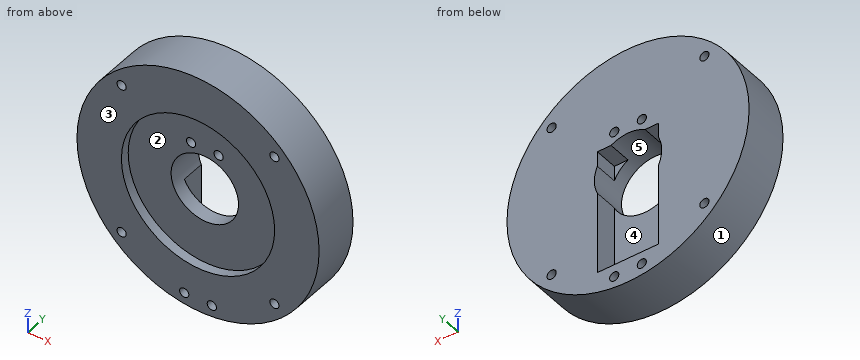
from build123d import *

# Parameters (mm, degrees)
CROQUIS1_R              = 39.5
CROQUIS1_R_2            = 11
CROQUIS1_R_3            = 1.5
SALIENTE_EXTRUIR2_DEPTH = 15
CROQUIS2_R              = 1.5
CROQUIS2_W              = 20
CROQUIS2_H              = 41
CORTAR_EXTRUIR1_DEPTH   = 7.5
CROQUIS2_2_R            = 1.5
CORTAR_EXTRUIR2_DEPTH   = 16
CROQUIS3_R              = 25
CORTAR_EXTRUIR3_DEPTH   = 3


with BuildPart() as part:
    # Croquis1 → Saliente-Extruir2 (new body)
    with BuildSketch(Plane(origin=(0, 0, 0), x_dir=(1, 0, 0), z_dir=(0, 1, 0))):
        Circle(CROQUIS1_R)
        Circle(CROQUIS1_R_2, mode=Mode.SUBTRACT)
        with Locations((24.925514037, 24.925514037)):
            Circle(CROQUIS1_R_3, mode=Mode.SUBTRACT)
        with Locations((24.925514037, -24.925514037)):
            Circle(CROQUIS1_R_3, mode=Mode.SUBTRACT)
        with Locations((-24.925514037, -24.925514037)):
            Circle(CROQUIS1_R_3, mode=Mode.SUBTRACT)
        with Locations((-24.925514037, 24.925514037)):
            Circle(CROQUIS1_R_3, mode=Mode.SUBTRACT)
    extrude(amount=SALIENTE_EXTRUIR2_DEPTH)

    # Croquis2 → Cortar-Extruir1 (cut)
    with BuildSketch(Plane(origin=(0, 15, 0), x_dir=(1, 0, 0), z_dir=(0, 1, 0))):
        with Locations((-4.5, -13.5)):
            Circle(CROQUIS2_R)
        with Locations((4.5, -13.5)):
            Circle(CROQUIS2_R)
        with Locations((4.5, 35.5)):
            Circle(CROQUIS2_R)
        with Locations((-4.5, 35.5)):
            Circle(CROQUIS2_R)
        with Locations((0, 11)):
            Rectangle(CROQUIS2_W, CROQUIS2_H)
    extrude(amount=-CORTAR_EXTRUIR1_DEPTH, mode=Mode.SUBTRACT)

    # Croquis2<2> → Cortar-Extruir2 (cut, through all)
    with BuildSketch(Plane(origin=(0, 15, 0), x_dir=(1, 0, 0), z_dir=(0, 1, 0))):
        with Locations((-4.5, 35.5)):
            Circle(CROQUIS2_2_R)
        with Locations((4.5, 35.5)):
            Circle(CROQUIS2_2_R)
        with Locations((4.5, -13.5)):
            Circle(CROQUIS2_2_R)
        with Locations((-4.5, -13.5)):
            Circle(CROQUIS2_2_R)
    extrude(amount=-CORTAR_EXTRUIR2_DEPTH, mode=Mode.SUBTRACT)

    # Croquis3 → Cortar-Extruir3 (cut)
    with BuildSketch(Plane.XZ):
        Circle(CROQUIS3_R)
    extrude(amount=-CORTAR_EXTRUIR3_DEPTH, mode=Mode.SUBTRACT)


solid = part.part
The listing builds one solid part. Answer for the finished solid, in the listing's coordinates (mm). Face numbers are marked on the shaded views. A direction names the side the tool comes from. Coordinates: 2 decimals unless noted, no trailing zeros. Write each loop counter-clockwise with the first axis right and the second up, starting at its lowest first coordinate (ties: lowest second). Pieces come first, ordered by that corner, then holes. Notation, with made-up numbers: (12.5, -15.75) -> (66.5, -15.75) arc R21 ccw to (66.5, 6.25) -> close; hole circle Ø10 at (-27, 5.25). An arc over 180 degrees is marked (long way). One line per question, with ' | ' between items.
1. Section D-D (y = 10) is taken. State how many separate pieces and enclosed holes the cut face has, and give its area (3 significant figures).
Verdict:
separate pieces: 1 | enclosed holes: 9 | area: 4,000 mm^2
2. Section C-C (z = 13.5) is taken. Determine the outline of the cut face in (x, y).
Verdict:
outline: (-37.12, 0) -> (-21.04, 0) -> (-21.04, 3) -> (-6, 3) -> (-6, 15) -> (-37.12, 15) -> close; (-3, 3) -> (3, 3) -> (3, 15) -> (-3, 15) -> close; (6, 3) -> (21.04, 3) -> (21.04, 0) -> (37.12, 0) -> (37.12, 15) -> (6, 15) -> close
3. Which of the six approach directions +Z, -Z, +X, -X, +Y, -Y give full straight-line access (tool end or side, diameter ignored) to the marked faces 4 and 5?
Verdict:
face 4: +Y | face 5: +Y, -Y
4. For a pull along X with two mould halves and no side action, classify the marked faces 1, 2 and 3 as released by +X, released by -X, zero draft, split by the parting line, or undercut.
Verdict:
face 1: split by the parting line | face 2: undercut | face 3: zero draft
5. Straight lines are drawn through the part: line 1 (Z direction, x = 0, y = 11.75); line 2 (Z direction, x = 4.5, y = 9.5); line 3 (X direction, y = 13.5, z = 0). For each, find the intervals that lie inside material, in ascending order.
Verdict:
line 1: z = -39.5 to -31.5, 11 to 39.5 | line 2: z = -39.24 to -37, -34 to -31.5, 10.04 to 12, 15 to 39.24 | line 3: x = -39.5 to -11, 11 to 39.5
6. Section A-A (z = 0) is taken. Determine the outline of the cut face in (x, y).
Verdict:
outline: (-39.5, 0) -> (-25, 0) -> (-25, 3) -> (-11, 3) -> (-11, 15) -> (-39.5, 15) -> close; (11, 3) -> (25, 3) -> (25, 0) -> (39.5, 0) -> (39.5, 15) -> (11, 15) -> close
7. Given pin 1 Ø2 at (x, y) = (-10.5, 4) entering from -Z; pin 2 Ø5 at (x, y) = (-7.5, 12.5) entering from -Z; pin 3 Ø4 at (x, z) = (10.5, 8) entering from -Y, each flat-ended and moving along its own axis, determine where each tip first touches the part or whether it passes through.
Verdict:
pin 1: stops at z = -38.34 | pin 2: stops at z = -39.18 | pin 3: stops at y = 3
8. Section B-B (x = 4.5) is taken. Determine the outline of the cut face in (y, z).
Verdict:
outline: (0, -39.24) -> (15, -39.24) -> (15, -37) -> (0, -37) -> close; (0, -34) -> (15, -34) -> (15, -31.5) -> (7.5, -31.5) -> (7.5, -10.04) -> (3, -10.04) -> (3, -24.59) -> (0, -24.59) -> close; (0, 24.59) -> (3, 24.59) -> (3, 15) -> (15, 15) -> (15, 39.24) -> (0, 39.24) -> close; (3, 10.04) -> (15, 10.04) -> (15, 12) -> (3, 12) -> close
